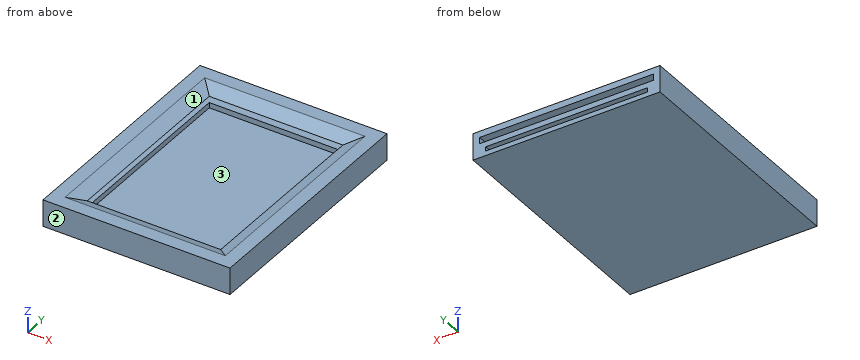
```python
from build123d import *

# Parameters (mm, degrees)
SKETCH1_W            = 88.9
SKETCH1_H            = 114.3
BOSS_EXTRUDE1_DEPTH  = 12.7
SKETCH2_W            = 76.835
SKETCH2_H            = 2.032
TOPLOADER_CUT_DEPTH  = 105.41
SKETCH3_W            = 63.5
SKETCH3_H            = 88.9
VIEWING_WINDOW_DEPTH = 9.525
CHAMFER1_SIZE        = 6.35
CHAMFER1_SIZE2       = 2.961053629
ACRYLIC_CUT_W        = 82.55
ACRYLIC_CUT_H        = 3
CUT_EXTRUDE1_DEPTH   = 109.22


with BuildPart() as part:
    # Sketch1 → Boss-Extrude1 (new body)
    with BuildSketch(Plane.XY):
        with Locations((44.45, 57.15)):
            Rectangle(SKETCH1_W, SKETCH1_H)
    extrude(amount=BOSS_EXTRUDE1_DEPTH)

    # Sketch2 → toploader_cut (cut)
    with BuildSketch(Plane(origin=(0, 114.3, 0), x_dir=(1, 0, 0), z_dir=(0, 1, 0))):
        with Locations((44.45, -3.175)):
            Rectangle(SKETCH2_W, SKETCH2_H)
    extrude(amount=-TOPLOADER_CUT_DEPTH, mode=Mode.SUBTRACT)

    # Sketch3 → viewing_window (cut)
    with BuildSketch(Plane.XY.offset(12.7)):
        with Locations((44.45, 57.15)):
            Rectangle(SKETCH3_W, SKETCH3_H)
    extrude(amount=-VIEWING_WINDOW_DEPTH, mode=Mode.SUBTRACT)

    # Chamfer1
    chamfer1_edges = [part.edges().sort_by_distance(p)[0] for p in [
        (12.7, 57.15, 12.7),
        (44.45, 12.7, 12.7),
        (76.2, 57.15, 12.7),
        (44.45, 101.6, 12.7),
    ]]
    chamfer1_side = [part.faces().sort_by_distance(p)[0] for p in [
        (44.45, 1.44802279, 12.7),
    ]]
    chamfer(chamfer1_edges, length=CHAMFER1_SIZE, length2=CHAMFER1_SIZE2, reference=chamfer1_side[0])

    # acrylic_cut → Cut-Extrude1 (cut)
    with BuildSketch(Plane(origin=(0, 114.3, 0), x_dir=(1, 0, 0), z_dir=(0, 1, 0))):
        with Locations((44.45, -8.238946371)):
            Rectangle(ACRYLIC_CUT_W, ACRYLIC_CUT_H)
    extrude(amount=-CUT_EXTRUDE1_DEPTH, mode=Mode.SUBTRACT)


solid = part.part
```
The model under review builds one solid part; all positions refer to its coordinate system, in mm. Face numbers are marked on the shaded views. Round coordinates to 2 decimals unless told otherwise and drop trailing zeros. Loops run counter-clockwise (first coordinate to the right, second up) from the corner with the lowest first, then second, coordinate; pieces in that order, holes last. Notation, with made-up numbers: (21, -38) -> (36, -38) arc R18 cw to (36, -12) -> close; hole circle Ø7 at (58.25, -20). An arc over 180 degrees is marked (long way). Answer as a JSON object with one key per item and string values. Group by question number.
1) We need section A-A on x = 32.5. Write out the cut boundary in (y, z), then the cut area to 3 significant figures.
2) We need section C-C on z = 11.25. Write out the cut boundary in (x, y).
3) For pin 1 Ø1 at (x, y) = (50, 35) entering from +Z; pin 2 Ø0.9 at (x, z) = (27.5, 8) entering from +Y; pin 3 Ø1 at (x, z) = (38.5, 3) entering from +Y, all flat-tipped, find the tip position at first contact; note any pin that passes through.
4) We need section D-D on y = 11.5. Give the number of separate pieces and of enclosed holes in the cut face, then the cut area to 3 significant figures.
5) Mouldability with a two-part tool opening along Y and no side actions: class the marked faces 1, 2 and 3 as released by +Y, released by -Y, zero draft, split by the parting line, or undercut.
6) For line 1 (Y direction, x = 71, z = 5.25); line 2 (X direction, y = 105.5, z = 7.5) (3 decimals); line 3 (Z direction, x = 12, y = 68.5), list the stretches that pass through material, from the lowest coordinate up. Write a range as [from, to].
Result set:
{
 "1": {"outline": "(0, 0) -> (114.3, 0) -> (114.3, 2.16) -> (8.89, 2.16) -> (8.89, 4.19) -> (12.7, 4.19) -> (12.7, 6.74) -> (5.08, 6.74) -> (5.08, 9.74) -> (12.7, 9.74) -> (6.35, 12.7) -> (0, 12.7) -> close; (101.6, 4.19) -> (114.3, 4.19) -> (114.3, 6.74) -> (101.6, 6.74) -> close; (101.6, 9.74) -> (114.3, 9.74) -> (114.3, 12.7) -> (107.95, 12.7) -> close", "area": "401 mm²"},
 "2": {"outline": "(0, 0) -> (88.9, 0) -> (88.9, 114.3) -> (0, 114.3) -> close; hole (9.46, 9.46) -> (79.44, 9.46) -> (79.44, 104.84) -> (9.46, 104.84) -> close"},
 "3": {"pin 1": "z = 2.16", "pin 2": "y = 5.08", "pin 3": "y = 8.89"},
 "4": {"separate pieces": "1", "enclosed holes": "2", "area": "555 mm²"},
 "5": {"face 1": "undercut", "face 2": "released by -Y", "face 3": "zero draft"},
 "6": {"line 1": "[0, 12.7], [101.6, 114.3]", "line 2": "[0, 3.175], [85.725, 88.9]", "line 3": "[0, 2.16], [4.19, 6.74], [9.74, 10.07]"}
}
